Can you work these out from the model? Positions are in its coordinate system, mm. A direction names the side the tool comes from. Coordinates: 2 decimals unless noted, no trailing zeros. Loops run counter-clockwise (first coordinate to the right, second up) from the corner with the lowest first, then second, coordinate; pieces in that order, holes last.
```python
from build123d import *

# Parameters (mm, degrees)
F0_R     = 78.013982
F1_DEPTH = 25.4
F2_R     = 9.510574
F3_DEPTH = 25.401
F5_DEPTH = 25.401
F7_DEPTH = 25.401


with BuildPart() as f1:
    # F0 (on Top) → F1 (new body)
    with BuildSketch(Plane.XY):
        Circle(F0_R)
    extrude(amount=F1_DEPTH)

    # F2 (on face) → F3 (cut, through all)
    with BuildSketch(Plane.XY.offset(25.4)):
        Circle(F2_R)
    extrude(amount=-F3_DEPTH, mode=Mode.SUBTRACT)

    # F4 (on face) → F5 (cut, through all)
    with BuildSketch(Plane(origin=(0, 0, 0), x_dir=(1, 0, 0), z_dir=(0, 0, -1))):
        with BuildLine():
            ThreePointArc((33.933129, -52.977759), (60.378444, 17.678906), (0, 62.913434))
            ThreePointArc((0, 62.913434), (-8.519115, 54.39432), (0, 45.875205))
            ThreePointArc((0, 45.875205), (44.026741, 12.891101), (24.743352, -38.630312))
            ThreePointArc((24.743352, -38.630312), (22.164517, -50.398924), (33.933129, -52.977759))
        make_face()
    extrude(amount=-F5_DEPTH, mode=Mode.SUBTRACT)

    # F6 (on face) → F7 (cut, through all)
    with BuildSketch(Plane.XY.offset(25.4)):
        with BuildLine():
            ThreePointArc((-24.743352, -38.630312), (-44.026741, 12.891101), (0, 45.875205))
            ThreePointArc((0, 45.875205), (8.519115, 54.39432), (0, 62.913434))
            ThreePointArc((0, 62.913434), (-60.378444, 17.678906), (-33.933129, -52.977759))
            ThreePointArc((-33.933129, -52.977759), (-22.164517, -50.398924), (-24.743352, -38.630312))
        make_face()
    extrude(amount=-F7_DEPTH, mode=Mode.SUBTRACT)


solid = f1.part
```
Item 1: On a 3-axis mill with a long thin cutter (end or side, diameter ignored), from which of +Z, -Z, +X, -X, +Y, -Y can I reach the whole of each face in a straight line? I mean faces 1 (the face through (16, 1, 0)), 2 (the face through (-8.517, -54.582, 12.522)). Say none if no direction works.
Results are:
face 1: -Z, +X, -X, +Y, -Y
face 2: +Z, -Z
Item 2: We'd pull the mould along Y, two halves only. Please class faces 3 (the face through (-77.94, 3.43, 12.52)), 4 (the face through (16, 1, 25.4)), 5 (the face through (-7.547, -5.787, 12.878)): +Y half, -Y half, draft (parallel to the pull), parting line (faces both ways), or undercut.
Results are:
face 3: parting line
face 4: draft
face 5: undercut
Item 3: I'm going to push flat-ended pins straight in: P1, Ø5, axis at x = -30, y = -58.5, coming from the -Z side; P2, Ø1, axis at x = -39, z = 10, coming from the +Y side; P3, Ø8, axis at x = -46.5, z = 3.5, coming from the -Y side; P4, Ø4, axis at x = 13.5, z = 3.5, coming from the +Y side. Where does each tip first touch, or does it pass through?
Results are:
P1: stops at z = 0
P2: stops at y = 67.85
P3: stops at y = -65.42
P4: stops at y = 77.16
Item 4: Suppose I cut it at B-B, the plane x = -58. Please give me the cut outline in (y, z), plus the area to 3 significant figures.
Results are:
outline: (-52.17, 0) - (-24.37, 0) - (-24.37, 25.4) - (-52.17, 25.4) - close; (24.37, 0) - (52.17, 0) - (52.17, 25.4) - (24.37, 25.4) - close
area: 1,410 mm2
Item 5: Suppose I cut it at C-C, the plane y = -36. Please give me the cut outline in (x, z).
Results are:
outline: (-69.21, 0) - (-51.6, 0) - (-51.6, 25.4) - (-69.21, 25.4) - close; (-28.43, 0) - (28.43, 0) - (28.43, 25.4) - (-28.43, 25.4) - close; (51.6, 0) - (69.21, 0) - (69.21, 25.4) - (51.6, 25.4) - close
Item 6: Suppose I cut it at D-D, the plane z = 23.25. Please give me the cut outline in (x, y).
Results are:
outline: circle Ø156.03 at (0, 0); hole (-33.93, -52.98) arc R8.52 ccw to (-24.74, -38.63) arc R45.88 cw to (0, 45.88) arc R8.52 ccw to (0, 62.91) arc R62.91 ccw to start; hole circle Ø19.02 at (0, 0); hole (0, -62.91) arc R62.91 ccw to (33.93, 52.98) arc R8.52 ccw to (24.74, 38.63) arc R45.88 cw to (0, -45.88) arc R8.52 ccw to start
Item 7: I need wall thicknesses on line 1 along X through (y, z) = (-1.5, 4.75); line 2 along Y through (x, z) = (34, 13.5); line 3 along X through (y, z) = (-37.5, 5.75). Which ranges of each line are inside material? Lowest first, please.
Results are:
line 1: x = -78 to -62.9, -45.85 to -9.39, 9.39 to 45.85, 62.9 to 78
line 2: y = -70.22 to -52.93, -30.8 to 30.8, 52.93 to 70.22
line 3: x = -68.41 to -50.52, -26.43 to 26.43, 50.52 to 68.41
Item 8: Suppose I cut it at A-A, the plane y = 0. Please give me the cut outline in (x, z).
Results are:
outline: (-78.01, 0) - (-62.91, 0) - (-62.91, 25.4) - (-78.01, 25.4) - close; (-45.88, 0) - (-9.51, 0) - (-9.51, 25.4) - (-45.88, 25.4) - close; (9.51, 0) - (45.88, 0) - (45.88, 25.4) - (9.51, 25.4) - close; (62.91, 0) - (78.01, 0) - (78.01, 25.4) - (62.91, 25.4) - close
